from build123d import *

# Parameters (mm, degrees)
SKETCH_R        = 2
PAD_DEPTH       = 4
SKETCH001_W     = 50
SKETCH001_H     = 3
PAD001_DEPTH    = 4
SKETCH002_R     = 2
PAD002_DEPTH    = 11
SKETCH003_W     = 57.312547
SKETCH003_H     = 35.48627
SKETCH003_W_2   = 32.934865
SKETCH003_H_2   = 4.062765
POCKET_DEPTH    = 11.001
SKETCH004_W     = 47.141797
SKETCH004_H     = 11.210097
POCKET001_DEPTH = 18.965808


with BuildPart() as part:
    # Sketch → Pad (new body)
    with BuildSketch(Plane.XY):
        with BuildLine():
            Line((10, 0), (40, 0))
            ThreePointArc((40, 0), (47.071068, 2.928932), (50, 10))
            Line((50, 10), (50, 22))
            Line((50, 22), (0, 22))
            Line((0, 22), (0, 10))
            ThreePointArc((0, 10), (2.928932, 2.928932), (10, 0))
        make_face()
        with Locations((7, 19)):
            Circle(SKETCH_R, mode=Mode.SUBTRACT)
        with Locations((31, 19)):
            Circle(SKETCH_R, mode=Mode.SUBTRACT)
    extrude(amount=PAD_DEPTH)

    # Sketch001 → Pad001 (join)
    with BuildSketch(Plane.XY):
        with Locations((25, 23.5)):
            Rectangle(SKETCH001_W, SKETCH001_H)
    extrude(amount=PAD001_DEPTH)

    # Sketch002 → Pad002 (join)
    with BuildSketch(Plane.XY):
        with BuildLine():
            Line((50, 11), (50, 22))
            Line((50, 22), (35, 22))
            ThreePointArc((35, 22), (31, 24), (27, 22))
            Line((27, 22), (11, 22))
            ThreePointArc((11, 22), (7, 24), (3, 22))
            Line((3, 22), (0, 22))
            Line((0, 22), (0, 11))
            Line((0, 11), (50, 11))
        make_face()
        with Locations((7, 19)):
            Circle(SKETCH002_R, mode=Mode.SUBTRACT)
        with Locations((31, 19)):
            Circle(SKETCH002_R, mode=Mode.SUBTRACT)
    extrude(amount=PAD002_DEPTH)

    # Sketch003 → Pocket (cut, through all)
    with BuildSketch(Plane.XY):
        with Locations((25.477233, 12.877207)):
            Rectangle(SKETCH003_W, SKETCH003_H)
        with Locations((19.127612, 16.933425)):
            Rectangle(SKETCH003_W_2, SKETCH003_H_2, mode=Mode.SUBTRACT)
    extrude(amount=POCKET_DEPTH, mode=Mode.SUBTRACT)

    # Sketch004 → Pocket001 (cut, through all)
    with BuildSketch(Plane.XZ):
        with Locations((17.359044, 8.036307)):
            Rectangle(SKETCH004_W, SKETCH004_H)
    extrude(amount=-POCKET001_DEPTH, mode=Mode.SUBTRACT)


solid = part.part
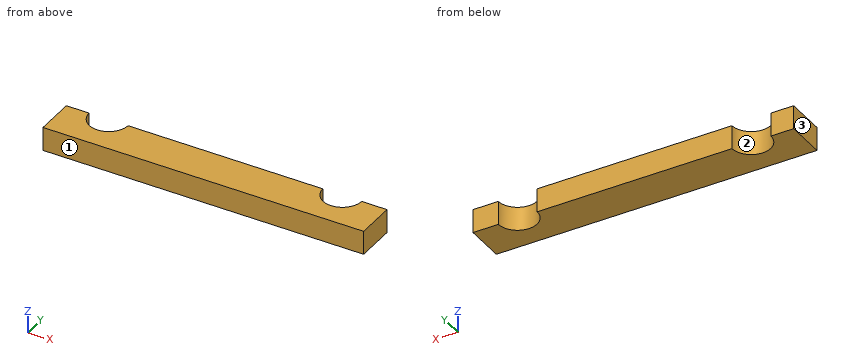
Model file for the job. Use its own axes, mm. Face numbers are marked on the shaded views. Coordinates: 2 decimals unless noted, no trailing zeros. Write each loop counter-clockwise with the first axis right and the second up, starting at its lowest first coordinate (ties: lowest second). Pieces come first, ordered by that corner, then holes. Notation, with made-up numbers: (9, 1) -> (15, 1) arc R26 ccw to (15, 39) -> close; hole circle Ø6 at (53, 75). An arc over 180 degrees is marked (long way). One line per item, written item: value. Start each with the question number.
1) Slice it at D-D on x = 32. Write the cut outline in (y, z), then the cut area to 3 significant figures.
2) Slice it at A-A on y = 18.3. Write the cut outline in (x, z), then the cut area to 3 significant figures.
3) Pull direction X, two halves, no side cores. Call the marked faces 1, 2 and 3: +X half, -X half, draft (parallel to the pull), parting line (faces both ways), or undercut.
4) Slice it at C-C on x = 7. Write the cut outline in (y, z).
5) Slice it at B-B on z = 0.65. Write the cut outline in (x, y).
6) Probe probe 1 along X at (y, z) = (17.45, 0.3); probe 2 along X at (y, z) = (18.5, 0.25); probe 3 along Y at (x, z) = (7, 1.7). List the from-to ranges inside material, lowest first.
Answers follow:
1. outline: (14.9, 0) -> (17.27, 0) -> (17.27, 2.43) -> (14.9, 2.43) -> close
1. area: 5.75 mm2
2. outline: (2.66, 0) -> (5.13, 0) -> (5.13, 2.43) -> (2.66, 2.43) -> close; (8.87, 0) -> (29.13, 0) -> (29.13, 2.43) -> (8.87, 2.43) -> close; (32.87, 0) -> (35.6, 0) -> (35.6, 2.43) -> (32.87, 2.43) -> close
2. area: 61.9 mm2
3. face 1: draft
3. face 2: undercut
3. face 3: -X half
4. outline: (14.9, 0) -> (17, 0) -> (17, 2.43) -> (14.9, 2.43) -> close
5. outline: (2.66, 14.9) -> (35.6, 14.9) -> (35.6, 18.96) -> (33, 18.96) arc R2 cw to (29, 18.96) -> (9, 18.96) arc R2 cw to (5, 18.96) -> (2.66, 18.96) -> close
6. probe 1: 2.66 to 5.74, 8.26 to 29.74, 32.26 to 35.6
6. probe 2: 2.66 to 5.06, 8.94 to 29.06, 32.94 to 35.6
6. probe 3: 14.9 to 17
